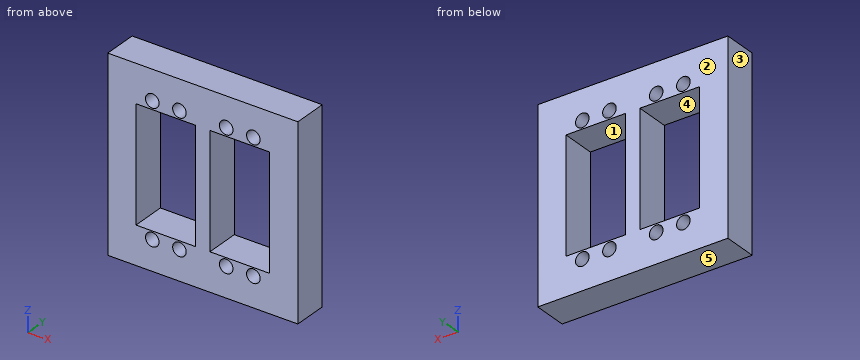
```python
from build123d import *

# Parameters (mm, degrees)
SKETCH1_W           = 70
SKETCH1_H           = 70
SKETCH1_R           = 2.5
SKETCH1_W_2         = 22
SKETCH1_H_2         = 42
BOSS_EXTRUDE1_DEPTH = 12.5


with BuildPart() as part:
    # Sketch1 → Boss-Extrude1 (new body)
    with BuildSketch(Plane(origin=(0, 0, 0), x_dir=(1, 0, 0), z_dir=(0, 1, 0))):
        Rectangle(SKETCH1_W, SKETCH1_H)
        with Locations(Location((-18.608500965, 24, 0), (0, 0, 270))):
            Circle(SKETCH1_R, mode=Mode.SUBTRACT)
        with Locations(Location((-8.608500965, 24, 0), (0, 0, 270))):
            Circle(SKETCH1_R, mode=Mode.SUBTRACT)
        with Locations(Location((-8.608500965, -24, 0), (0, 0, 90))):
            Circle(SKETCH1_R, mode=Mode.SUBTRACT)
        with Locations(Location((-18.608500965, -24, 0), (0, 0, 90))):
            Circle(SKETCH1_R, mode=Mode.SUBTRACT)
        with Locations(Location((8.608500965, -24, 0), (0, 0, 270))):
            Circle(SKETCH1_R, mode=Mode.SUBTRACT)
        with Locations(Location((18.608500965, -24, 0), (0, 0, 270))):
            Circle(SKETCH1_R, mode=Mode.SUBTRACT)
        with Locations(Location((8.608500965, 24, 0), (0, 0, 90))):
            Circle(SKETCH1_R, mode=Mode.SUBTRACT)
        with Locations(Location((18.608500965, 24, 0), (0, 0, 90))):
            Circle(SKETCH1_R, mode=Mode.SUBTRACT)
        with Locations((-13.608500965, 0)):
            Rectangle(SKETCH1_W_2, SKETCH1_H_2, mode=Mode.SUBTRACT)
        with Locations((13.608500965, 0)):
            Rectangle(SKETCH1_W_2, SKETCH1_H_2, mode=Mode.SUBTRACT)
    extrude(amount=BOSS_EXTRUDE1_DEPTH)


solid = part.part
```
For this review, take the finished solid that the model builds, in its own axes (mm). Face numbers are marked on the shaded views. A direction names the side the tool comes from. Coordinates: 2 decimals unless noted, no trailing zeros. Order: outer loops, then holes, each group sorted by start corner. A loop starts at its lowest first (then second) coordinate and runs counter-clockwise, first axis right, second up. Notation, with made-up numbers: (56, 37) -> (72, 37) arc R11 ccw to (72, 43) -> close; hole circle Ø1 at (14, 24). An arc over 180 degrees is marked (long way). Use CSV: the item, a comma, the result in double quotes. Start each with the question number.
Item 1: We need section D-D, the plane x = -7. Give the boundary of the cut face in (y, z), then the cut area to 3 significant figures.
Item 2: We need section C-C, the plane z = -11.5. Give the boundary of the cut face in (x, y), then the cut area to 3 significant figures.
Item 3: Draft analysis for pull direction X (two halves, no side actions). For the marked faces 3, 4 and 5, state which applies: pulls with the +X half, pulls with the -X half, needs draft (parallel to the pull), parting line crosses it, or undercut.
Item 4: We need section B-B, the plane x = 4.5. Give the boundary of the cut face in (y, z).
Item 5: Insertion check: pin 1 (4 mm diameter, centred on x = 18.61, z = -24, fed in from -Y); pin 2 (6.5 mm diameter, centred on x = -18.61, z = -24, fed in from +Y). Each pin has a flat end and moves straight along its axis. Give the tip position at first contact, or say it passes through.
Item 6: For the marked faces 1 and 2, list the 3-axis set-ups (+Z, -Z, +X, -X, +Y, -Y) from which the entire face can be reached by the end or side of a thin tool; tool diameter is ignored.
Item 7: Wall thickness on probe 1 along X at (y, z) = (5.5, 24); probe 2 along Z at (x, y) = (-18.5, 8.75); probe 3 along X at (y, z) = (3.5, 1): over which ranges is each line inside the solid? List them lowest first.
Item 8: We need section A-A, the plane z = -24. Give the boundary of the cut face in (x, y), then the cut area to 3 significant figures.
Derived:
1,outline,"(0, -35) -> (12.5, -35) -> (12.5, -25.91) -> (0, -25.91) -> close; (0, -22.09) -> (12.5, -22.09) -> (12.5, -21) -> (0, -21) -> close; (0, 21) -> (12.5, 21) -> (12.5, 22.09) -> (0, 22.09) -> close; (0, 25.91) -> (12.5, 25.91) -> (12.5, 35) -> (0, 35) -> close"
1,area,"254 mm^2"
2,outline,"(-35, 0) -> (-24.61, 0) -> (-24.61, 12.5) -> (-35, 12.5) -> close; (-2.61, 0) -> (2.61, 0) -> (2.61, 12.5) -> (-2.61, 12.5) -> close; (24.61, 0) -> (35, 0) -> (35, 12.5) -> (24.61, 12.5) -> close"
2,area,"325 mm^2"
3,face 3,"pulls with the -X half"
3,face 4,"undercut"
3,face 5,"needs draft"
4,outline,"(0, -35) -> (12.5, -35) -> (12.5, -21) -> (0, -21) -> close; (0, 21) -> (12.5, 21) -> (12.5, 35) -> (0, 35) -> close"
5,pin 1,"passes through"
5,pin 2,"stops at y = 12.5"
6,face 1,"+Y, -Y"
6,face 2,"+Z, -Z, +X, -X, +Y"
7,probe 1,"x = -35 to -21.11, -16.11 to -11.11, -6.11 to 6.11, 11.11 to 16.11, 21.11 to 35"
7,probe 2,"z = -35 to -26.5, -21.5 to -21, 21 to 21.5, 26.5 to 35"
7,probe 3,"x = -35 to -24.61, -2.61 to 2.61, 24.61 to 35"
8,outline,"(-35, 0) -> (-21.11, 0) -> (-21.11, 12.5) -> (-35, 12.5) -> close; (-16.11, 0) -> (-11.11, 0) -> (-11.11, 12.5) -> (-16.11, 12.5) -> close; (-6.11, 0) -> (6.11, 0) -> (6.11, 12.5) -> (-6.11, 12.5) -> close; (11.11, 0) -> (16.11, 0) -> (16.11, 12.5) -> (11.11, 12.5) -> close; (21.11, 0) -> (35, 0) -> (35, 12.5) -> (21.11, 12.5) -> close"
8,area,"625 mm^2"
